The model under review builds one solid part; all positions refer to its coordinate system, in mm. A direction names the side the tool comes from. Coordinates: 2 decimals unless noted, no trailing zeros.
```python
from build123d import *

# Parameters (mm, degrees)
F0_W     = 120
F0_H     = 194
F1_DEPTH = 12
F3_D     = 6
F3_DEPTH = 30
F3_TIP   = 1.8025818571
F5_D     = 6
F5_DEPTH = 30
F5_TIP   = 1.8025818571


with BuildPart() as f1:
    # F0 (on Front) → F1 (new body)
    with BuildSketch(Plane.XZ):
        Rectangle(F0_W, F0_H)
    extrude(amount=F1_DEPTH)

    # F3
    with Locations(Plane.XY.offset(97)):
        with Locations((-50, -6), (0, -6), (50, -6)):
            Hole(F3_D / 2, depth=F3_DEPTH)
            with Locations((0, 0, -(F3_DEPTH + F3_TIP / 2))):  # 118° drill point
                Cone(0, F3_D / 2, F3_TIP, mode=Mode.SUBTRACT)

    # F5
    with Locations(Plane(origin=(0, 0, -97), x_dir=(1, 0, 0), z_dir=(0, 0, -1))):
        with Locations((-50, 6), (0, 6), (50, 6)):
            Hole(F5_D / 2, depth=F5_DEPTH)
            with Locations((0, 0, -(F5_DEPTH + F5_TIP / 2))):  # 118° drill point
                Cone(0, F5_D / 2, F5_TIP, mode=Mode.SUBTRACT)


solid = f1.part
```
(1) For pin 1 Ø3.5 at (x, y) = (50, -6) entering from +Z; pin 2 Ø3.5 at (x, y) = (0, -6) entering from -Z; pin 3 Ø5 at (x, y) = (-50, -6) entering from +Z, all flat-tipped, find the tip position at first contact; note any pin that passes through.
A:
pin 1: stops at z = 66.25
pin 2: stops at z = -66.25
pin 3: stops at z = 66.7
(2) Draft analysis for pull direction Y (two halves, no side actions). For faces 1 (the face through (-1, -2, 97)), 2 (the face through (0, -3, 82)), 3 (the face through (-1, -12, 1)), 4 (the face through (-47, -6, -82)), state which applies: released by +Y, released by -Y, zero draft, split by the parting line, or undercut.
A:
face 1: zero draft
face 2: undercut
face 3: released by -Y
face 4: undercut
(3) Machinability: for faces 5 (the face through (53, -6, 82)), 6 (the face through (-60, -6, -1)), 7 (the face through (0.65, -3.07, -81.79)), which of the approach directions +Z, -Z, +X, -X, +Y, -Y give a long, thin tool a straight path to every point of the face, cutting with its end or side? Answer none if there is none.
A:
face 5: +Z
face 6: +Z, -Z, -X, +Y, -Y
face 7: -Z
(4) Wall thickness on probe 1 along X at (y, z) = (-6, 86); probe 2 along Y at (x, z) = (0, -78.5); probe 3 along Z at (x, y) = (0, -5.25): over which ranges is each line inside the solid? List them lowest first.
A:
probe 1: x = -60 to -53, -47 to -3, 3 to 47, 53 to 60
probe 2: y = -12 to -9, -3 to 0
probe 3: z = -65.65 to 65.65
